Verification items for the finished model (mm, model axes). Face numbers are marked on the shaded views. A direction names the side the tool comes from. Round coordinates to 2 decimals unless told otherwise and drop trailing zeros. Write each loop counter-clockwise with the first axis right and the second up, starting at its lowest first coordinate (ties: lowest second). Pieces come first, ordered by that corner, then holes. Notation, with made-up numbers: (43, -5.75) - (67, -5.75) arc R5 cw to (67, -0.75) - close; hole circle Ø10 at (2.5, 23). An arc over 180 degrees is marked (long way). Write each question's results on one line, items separated by ' | '.
```python
from build123d import *

# Parameters (mm, degrees)
SKETCH1_R             = 30
BOSS_EXTRUDE1_DEPTH   = 50
SKETCH2_R             = 50
BOSS_EXTRUDE2_DEPTH   = 30
BOSS_EXTRUDE3_DEPTH   = 10
F_1_5MM_DOWEL_HOLE1_D = 30
CUT_EXTRUDE1_DEPTH    = 202.15131476


with BuildPart() as part:
    # Sketch1 → Boss-Extrude1 (new, symmetric)
    with BuildSketch(Plane.XY):
        Circle(SKETCH1_R)
    extrude(amount=BOSS_EXTRUDE1_DEPTH, both=True)



with BuildPart() as body_2:
    # Sketch2 → Boss-Extrude2 (new body)
    with BuildSketch(Plane.XY):
        with Locations((81.003249692, -80)):
            Circle(SKETCH2_R)
    extrude(amount=BOSS_EXTRUDE2_DEPTH)


with BuildPart() as part_1:
    add(part.part)

    add(body_2.part)  # Boss-Extrude3 merges body 2
    # Sketch3 → Boss-Extrude3 (add)
    with BuildSketch(Plane.XY):
        Polygon((17.003072039, 24.716301124), (109.34170309, -38.806164794), (45.716447378, -115.423743202), (-30, -40), (-30, 0), align=None)
    extrude(amount=BOSS_EXTRUDE3_DEPTH)

    # Ø1.5mm Dowel Hole1 (through all)
    with Locations(Plane.XY.offset(50)):
        with Locations((0, 0)):
            Hole(F_1_5MM_DOWEL_HOLE1_D / 2)

    # Sketch6 → Cut-Extrude1 (cut, through all)
    with BuildSketch(Plane.XY.offset(30)):
        with BuildLine():
            Line((111.003249692, -80), (111.003249692, -166.852911506))
            ThreePointArc((111.003249692, -166.852911506), (81.003249692, -196.852911506), (51.003249692, -166.852911506))
            Line((51.003249692, -166.852911506), (51.003249692, -80))
            ThreePointArc((51.003249692, -80), (81.003249692, -50), (111.003249692, -80))
        make_face()
    extrude(amount=-CUT_EXTRUDE1_DEPTH, mode=Mode.SUBTRACT)


solid = part_1.part
```
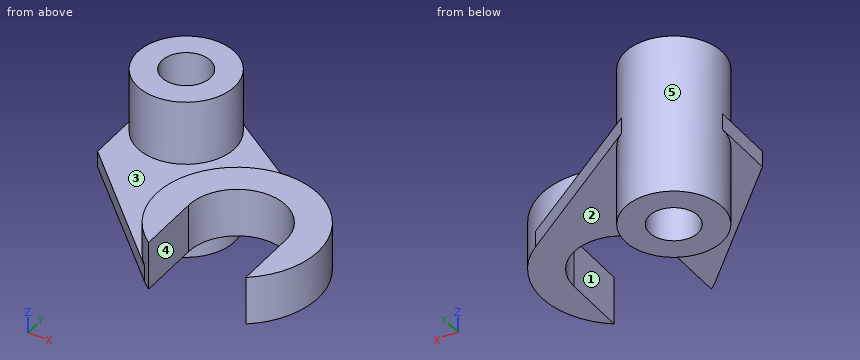
(1) Section check B-B (x = 0). Record the cut outline in (y, z), plus the area to 3 significant figures.
Answer:
outline: (-69.88, 0) - (-30, 0) - (-30, -50) - (-15, -50) - (-15, 50) - (-30, 50) - (-30, 10) - (-69.88, 10) - close; (15, -50) - (30, -50) - (30, 50) - (15, 50) - close | area: 3,400 mm2
(2) Go/stop test with flat-tipped pins: pin 1 Ø15 at (y, z) = (-96.5, 15.5) entering from -X; pin 2 Ø6 at (y, z) = (-72, 30.5) entering from +X; pin 3 Ø2 at (x, y) = (46.5, -42) entering from +Z. Record where each tip stops, or that it passes through.
Answer:
pin 1: x = 21.6 | pin 2: x = 130.75 | pin 3: z = 10
(3) Thickness scan on L1, parallel to X at y = -0.5, z = 15; L2, parallel to Y at x = 0, z = 27; L3, parallel to Y at x = -9.5, z = -7. Record the ranges inside material, lowest first.
Answer:
L1: -30 to -14.99, 14.99 to 30 | L2: -30 to -15, 15 to 30 | L3: -28.46 to -11.61, 11.61 to 28.46
(4) Section check A-A (z = 23). Record the cut outline in (x, y), plus the area to 3 significant figures.
Answer:
outline: circle Ø60 at (0, 0); (51, -120) - (51, -80) arc R30 cw to (111, -80) - (111, -120) arc R50 ccw (long way) to start; hole circle Ø30 at (0, 0) | area: 5,750 mm2
(5) Section check C-C (y = -10). Record the cut outline in (x, z).
Answer:
outline: (-30, 0) - (-28.28, 0) - (-28.28, -50) - (-11.18, -50) - (-11.18, 50) - (-28.28, 50) - (-28.28, 10) - (-30, 10) - close; (11.18, -50) - (28.28, -50) - (28.28, 0) - (67.47, 0) - (67.47, 10) - (28.28, 10) - (28.28, 50) - (11.18, 50) - close
(6) Set-up check for the marked faces 3, 4 and 5: record each of +Z, -Z, +X, -X, +Y, -Y from which the full face is reachable in a straight line by a thin tool's end or side.
Answer:
face 3: +Z | face 4: +Z, -Z, -Y | face 5: none
(7) Mould release check, pull along X, two halves, no side actions. Record for the marked faces 1 and 2: released by +X, released by -X, zero draft, split by the parting line, or undercut.
Answer:
face 1: undercut | face 2: zero draft
(8) Section check D-D (z = -2.5). Record the cut outline in (x, y).
Answer:
outline: circle Ø60 at (0, 0); hole circle Ø30 at (0, 0)
